```python
from build123d import *

# Parameters (mm, degrees)
BOSS_EXTRUDE1_DEPTH = 10
SKETCH2_W           = 25
SKETCH2_H           = 25
BOSS_EXTRUDE2_DEPTH = 5


with BuildPart() as part:
    # Sketch1 → Boss-Extrude1 (new body)
    with BuildSketch(Plane(origin=(0, 0, 0), x_dir=(0, 0, -1), z_dir=(1, 0, 0))):
        Polygon((0, 0), (0, 20), (5, 20), (5, -5), (-20, -5), (-20, 0), align=None)
    extrude(amount=BOSS_EXTRUDE1_DEPTH)

    # Sketch2 → Boss-Extrude2 (add)
    with BuildSketch(Plane(origin=(0, 0, 0), x_dir=(0, 0, -1), z_dir=(1, 0, 0))):
        with Locations((-7.5, 7.5)):
            Rectangle(SKETCH2_W, SKETCH2_H)
    extrude(amount=-BOSS_EXTRUDE2_DEPTH)


solid = part.part
```
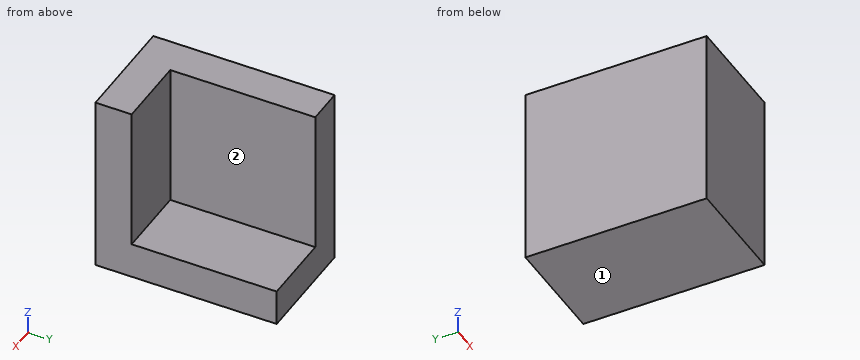
Input: part model. Units: mm. Frame: model coordinates. Face numbers are marked on the shaded views. A direction names the side the tool comes from. Coordinates: 2 decimals unless noted, no trailing zeros. Loops run counter-clockwise (first coordinate to the right, second up) from the corner with the lowest first, then second, coordinate; pieces in that order, holes last.
Q1. Contact query for flat-ended pins moving along their axis: pin 1 (6 mm diameter, centred on x = 5, z = 6, fed in from +Y); pin 2 (10 mm diameter, centred on y = 12.5, z = 13.5, fed in from +X); pin 3 (3 mm diameter, centred on x = 5, y = 8.5, fed in from +Z); pin 4 (8 mm diameter, centred on x = 2.5, y = 4, fed in from +Z). Output: stop coordinate, or through.
Results are:
pin 1: stops at y = 0
pin 2: stops at x = 0
pin 3: stops at z = 0
pin 4: stops at z = 20
Q2. Section A-A, the plane z = 4.25. Return the cut outline in (x, y), and give its area (3 significant figures).
Results are:
outline: (-5, -5) - (10, -5) - (10, 0) - (0, 0) - (0, 20) - (-5, 20) - close
area: 175 mm2
Q3. Line query: line 1 along Z through (x, y) = (6.5, 3.75). Output: solid intervals per line, ascending.
Results are:
line 1: z = -5 to 0
Q4. Section B-B, the plane x = 3.75. Return the cut outline in (y, z).
Results are:
outline: (-5, -5) - (20, -5) - (20, 0) - (0, 0) - (0, 20) - (-5, 20) - close
Q5. Set-up query: the marked faces 1 and 2. Return all of +Z, -Z, +X, -X, +Y, -Y with unobstructed straight access to the full face (end or side cutting, diameter ignored); none if empty.
Results are:
face 1: -Z, +X, -X, +Y, -Y
face 2: +Z, +X, +Y
